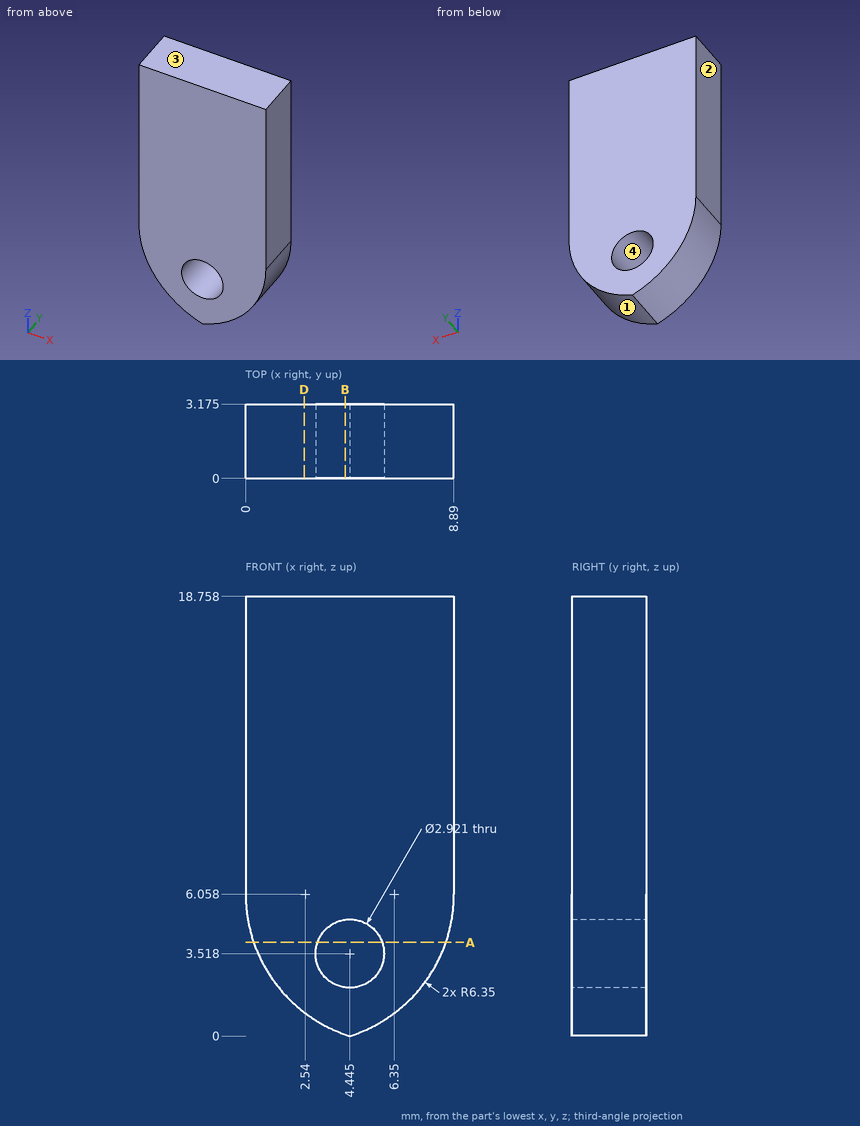
For this review, use the dimensioned drawing (mm, ordinates from the lowest corner) and the shaded views. Give positions to 0.01 mm unless a question says otherwise; leave off trailing zeros. Write each loop counter-clockwise with the first axis right and the second up, starting at its lowest first coordinate (ties: lowest second). Pieces come first, ordered by that corner, then holes. Notation, with made-up numbers: M -29.75,87.25 L 23.25,87.25 A3 cw 23.25,91.25 Z; hole C -18,68.25 d9. An arc over 180 degrees is marked long. Answer as a JSON object with one key per item and string values. Group by question number.
1) We need section A-A (z = 4). Give the boundary of the cut face in (x, y) (1 decimal), and give its area (3 significant figures).
2) We need section D-D (x = 2.5). Give the boundary of the cut face in (y, z) (1 decimal).
3) Mouldability with a two-part tool opening along Z and no side actions: class the marked faces 1, 2, 3 and 4 as released by +Z, released by -Z, zero draft, split by the parting line, or undercut.
4) We need section B-B (x = 4.25). Give the boundary of the cut face in (y, z) (1 decimal).
5) For line 1 along Z through (x, y) = (5.75, 0.6) (1 decimal); line 2 along Z through (x, y) = (5, 2.7) (1 decimal); line 3 along X through (y, z) = (0.7, 4.5) (1 decimal), list the stretches that pass through material, from the lowest coordinate up.
Answer key:
{
 "1": {"outline": "M 0.3,0 L 3.1,0 L 3.1,3.2 L 0.3,3.2 Z; M 5.8,0 L 8.5,0 L 8.5,3.2 L 5.8,3.2 Z", "area": "17.3 mm²"},
 "2": {"outline": "M 0,1 L 3.2,1 L 3.2,18.8 L 0,18.8 Z"},
 "3": {"face 1": "released by -Z", "face 2": "zero draft", "face 3": "released by +Z", "face 4": "undercut"},
 "4": {"outline": "M 0,0.1 L 3.2,0.1 L 3.2,2.1 L 0,2.1 Z; M 0,5 L 3.2,5 L 3.2,18.8 L 0,18.8 Z"},
 "5": {"line 1": "z = 0.6 to 2.9, 4.2 to 18.8", "line 2": "z = 0.2 to 2.2, 4.9 to 18.8", "line 3": "x = 0.2 to 3.4, 5.5 to 8.7"}
}
